Autodesk Inventor part; units mm, degrees
ref_plane "YZ Plane" through (0, 0, 0) normal (1, 0, 0) x (0, 1, 0)
ref_plane "XZ Plane" through (0, 0, 0) normal (0, 1, 0) x (-1, 0, 0)
ref_plane "XY Plane" through (0, 0, 0) normal (0, 0, 1) x (1, 0, 0)
sketch "Esboço1" plane through (0, 0, 0) normal (0, 1, 0) x (-1, 0, 0)
  line L0 (-1.2, -1.2) -> (-19.2, -1.2)
  line L1 (-19.2, -1.2) -> (-19.2, -6.2)
  line L2 (-19.2, -6.2) -> (-27.6, -6.2)
  line L3 (-27.6, -6.2) -> (-27.6, -1.2)
  line L4 (-27.6, -1.2) -> (-45.6, -1.2)
  line L5 (-45.6, -1.2) -> (-45.6, -6.2)
  arc A0 (-45.6, -6.2) -> (-1.2, -6.2) centre (-23.4, -6.2) ccw
  line L6 (-23.4, -6.2) -> (-45.6, -6.2) construction
  line L7 (-23.4, -6.2) -> (-1.2, -6.2) construction
  line L8 (-1.2, -6.2) -> (-1.2, -1.2)
  arc A1 (-46.8, -6.2) -> (0, -6.2) centre (-23.4, -6.2) ccw
  line L9 (0, -6.2) -> (0, 0)
  line L10 (0, 0) -> (-20.4, 0)
  line L11 (-20.4, 0) -> (-20.4, -5)
  line L12 (-20.4, -5) -> (-26.4, -5)
  line L13 (-46.8, 18) -> (-46.8, -6.2)
  line L14 (-27.6, -1.2) -> (-27.6, 18)
  line L15 (-19.2, -1.2) -> (-19.2, 0)
  line L16 (-1.2, -1.2) -> (-1.2, 0)
  arc A2 (-27.6, -6.2) -> (-19.2, -6.2) centre (-23.4, -6.2) ccw
  line L17 (-26.4, 18) -> (-46.8, 18)
  line L18 (-45.6, -1.2) -> (-45.6, 18)
  line L19 (-26.4, 18) -> (-26.4, -5)
  point P0 (-23.4, -6.2)
  point P1 (-46.8, -6.2)
  point P2 (-19.2, -6.2)
  point P3 (-27.6, -6.2)
  point P4 (-45.6, -6.2)
  point P5 (-36.6, 18)
  point P6 (-36.6, -1.2)
  point P7 (-45.6, -3.7)
  point P8 (-45.6, 8.4)
  point P9 (-23.4, -5)
  point P10 (-26.4, 6.5)
  dimension "d0" = 18
  dimension "d1" = 180
  dimension "d3" = 1.2
  dimension "d7" = 18
  dimension "d15" = 1.2
  dimension "d16" = 6
  dimension "d18" = 19.2
  dimension "d19" = 5
extrude "Extrusão1" add sketch "Esboço1" against normal blind 1.2
extrude "Extrusão3" add sketch "Esboço1" along normal blind 12.6 contours L16 L10 L9 A1 L13 L17 L18 L5 A0 L8 | L1 L2 L3 L14 L17 L19 L12 L11 L10 L15 | A2 L2
fillet "Arredondamento1" radius 9 6 edges at (1.2, 0, -3.1) (45.6, 0, 5.9) (23.4, 0, -28.4) (27.6, 0, 5.9) (19.2, 0, -3.1) (23.4, 0, -10.4)
equation "\"d0\" = Diâmetro_esfera"
equation "\"d3\" = Margem"
equation "\"d15\" = Margem"
equation "\"d16\" = Espessura_torre_base"
equation "\"d8\" = Margem"
equation "\"d12\" = 0.7 * Diâmetro_esfera"
equation "\"d14\" = 0.5 * Diâmetro_esfera"
equation "\"Diâmetro_esfera\" = 18"
equation "\"Filamento\" = 0.4"
equation "\"Margem\" = 3 * Filamento"
equation "\"Espessura_torre_base\" = 15 * Filamento"
properties part number "Troca de sentido" material "Plástico PET"
The model under review builds one solid part; all positions refer to its coordinate system, in mm. A direction names the side the tool comes from. Give positions to 0.01 mm unless a question says otherwise; leave off trailing zeros. Loops run counter-clockwise (first coordinate to the right, second up) from the corner with the lowest first, then second, coordinate; pieces in that order, holes last. Notation, with made-up numbers: (-36.75, -26.5) -> (-15.75, -26.5) arc R22 ccw to (-15.75, -10.5) -> close; hole circle Ø5 at (-21, 82.25). An arc over 180 degrees is marked (long way). Put each result on its own line as item: value. Start each with the question number.
1. Wall thickness on probe 1 along X at (y, z) = (9.5, 13.5); probe 2 along X at (y, z) = (4.5, -8.5); probe 3 along X at (y, z) = (11.25, -7): over which ranges is each line inside the solid? List them lowest first.
2. Clearance check with flat-ended pins moving along their axes: P1, Ø3, axis at y = 1, z = -5.5, coming from the -X side; P2, Ø4, axis at y = 11, z = 2.5, coming from the -X side; P3, Ø8, axis at y = 6, z = -16, coming from the +X side; P4, Ø1, axis at y = 9, z = -16.5, coming from the -X side. State where each tip first meets the part, or that it passes through.
3. Mouldability with a two-part tool opening along Z and no side actions: class faces 1 (the face through (23.3, 10.8, -10.4)), 2 (the face through (10.2, -0.4, 0)), 3 (the face through (3.906, 2.566, -3.143)) as released by +Z, released by -Z, zero draft, split by the parting line, or undercut.
4. For faces 4 (the face through (42.894, 2.566, 6.069)), 5 (the face through (0, 6, -3)), 6 (the face through (26.4, 6, 7)), list the 3-axis set-ups (+Z, -Z, +X, -X, +Y, -Y) from which the entire face can be reached by the end or side of a thin tool; tool diameter is ignored.
5. We need section A-A on y = 4.25. State the section outline as (x, z) points.
Determined:
1. probe 1: 26.4 to 27.6, 45.6 to 46.8
1. probe 2: 0.11 to 2.53, 18.51 to 28.29, 44.27 to 46.69
1. probe 3: 0.01 to 1.21, 19.28 to 27.52, 45.59 to 46.79
2. P1: x = 0
2. P2: x = 26.4
2. P3: x = 46.07
2. P4: x = 2.15
3. face 1: undercut
3. face 2: released by +Z
3. face 3: zero draft
4. face 4: +Z, +Y
4. face 5: +Z, -Z, -X, +Y, -Y
4. face 6: +Z, +Y, -Y
5. outline: (0, -6.2) arc R23.4 ccw to (46.8, -6.2) -> (46.8, 18) -> (44.24, 18) -> (44.24, -6.2) arc R20.84 cw to (2.56, -6.2) -> (2.56, 0) -> (0, 0) -> close; (17.84, -6.2) arc R5.56 ccw to (28.96, -6.2) -> (28.96, 18) -> (26.4, 18) -> (26.4, -5) -> (20.4, -5) -> (20.4, 0) -> (17.84, 0) -> close
